```python
from build123d import *

# Parameters (mm, degrees)
BOSS_EXTRUDE1_DEPTH = 31.75
SKETCH2_R           = 3.175
CUT_EXTRUDE1_DEPTH  = 4.175
SKETCH3_R           = 3.175
CUT_EXTRUDE2_DEPTH  = 4.175


with BuildPart() as part:
    # Sketch1 → Boss-Extrude1 (new body)
    with BuildSketch(Plane.XY):
        Polygon((0, 0), (0, 25.4), (3.175, 25.4), (3.175, 3.175), (38.1, 3.175), (38.1, 0), align=None)
    extrude(amount=BOSS_EXTRUDE1_DEPTH)

    # Sketch2 → Cut-Extrude1 (cut, through all)
    with BuildSketch(Plane(origin=(0, 3.175, 0), x_dir=(1, 0, 0), z_dir=(0, 1, 0))):
        with Locations((31.9786, -6.35)):
            Circle(SKETCH2_R)
        with Locations((31.9786, -25.4)):
            Circle(SKETCH2_R)
    extrude(amount=-CUT_EXTRUDE1_DEPTH, mode=Mode.SUBTRACT)

    # Sketch3 → Cut-Extrude2 (cut, through all)
    with BuildSketch(Plane(origin=(3.175, 0, 0), x_dir=(0, 0, -1), z_dir=(1, 0, 0))):
        with Locations((-25.4, 15.875)):
            Circle(SKETCH3_R)
        with Locations((-6.35, 15.875)):
            Circle(SKETCH3_R)
    extrude(amount=-CUT_EXTRUDE2_DEPTH, mode=Mode.SUBTRACT)


solid = part.part
```
Check sheet for the modelled part. Datum: model origin and axes. Units: mm. A direction names the side the tool comes from. Round coordinates to 2 decimals unless told otherwise and drop trailing zeros. Order: outer loops, then holes, each group sorted by start corner. A loop starts at its lowest first (then second) coordinate and runs counter-clockwise, first axis right, second up.
1) Tool access check on faces 5 (the flat face through (2, 25.4, 16)), 6 (the flat face through (3.175, 14, 16)). Record the directions out of +Z, -Z, +X, -X, +Y, -Y that give a thin tool (end or side, any length) a straight path to the whole face; none if there is none.
2) Section check C-C (y = 17). Record the boundary of the cut face in (x, z) (3 decimals), and give its area (3 significant figures).
3) Go/stop test with flat-tipped pins: pin 1 Ø6 at (y, z) = (5.5, 7) entering from -X; pin 2 Ø16 at (x, z) = (26, 20) entering from +Y (3 decimals); pin 3 Ø11 at (y, z) = (17, 22) entering from +X (3 decimals). Record where each tip stops, or that it passes through.
4) Section check D-D (z = 21.5). Record the boundary of the cut face in (x, y) (3 decimals).
5) Section check B-B (x = 30.5). Record the boundary of the cut face in (y, z) (3 decimals), and give its area (3 significant figures).
6) Section check A-A (z = 6.35). Record the boundary of the cut face in (x, y) (3 decimals), and give its area (3 significant figures).
7) Mould release check, pull along X, two halves, no side actions. Record for faces 1 (the cylindrical face through (34.91, 1.61, 7.57)), 2 (the flat face through (38.1, 2, 16)), 3 (the cylindrical face through (33.685, 1.61, 22.723)), 4 (the flat face through (20, 3.175, 16)): +X half, -X half, draft (parallel to the pull), parting line (faces both ways), or undercut.
8) Scan lines: line 1 (X direction, y = 1.05, z = 6.35); line 2 (Y direction, x = 1.35, z = 25.4); line 3 (X direction, y = 6.5, z = 18) (3 decimals). Record each from-to range of solid material in increasing order.
Result:
1. face 5: +Z, -Z, +X, -X, +Y
1. face 6: +Z, -Z, +X, +Y
2. outline: (0, 0) - (3.175, 0) - (3.175, 3.381) - (0, 3.381) - close; (0, 9.319) - (3.175, 9.319) - (3.175, 22.431) - (0, 22.431) - close; (0, 28.369) - (3.175, 28.369) - (3.175, 31.75) - (0, 31.75) - close
2. area: 63.1 mm2
3. pin 1: stops at x = 0
3. pin 2: stops at y = 3.175
3. pin 3: stops at x = 3.175
4. outline: (0, 0) - (38.1, 0) - (38.1, 3.175) - (3.175, 3.175) - (3.175, 25.4) - (0, 25.4) - close
5. outline: (0, 0) - (3.175, 0) - (3.175, 3.54) - (0, 3.54) - close; (0, 9.16) - (3.175, 9.16) - (3.175, 22.59) - (0, 22.59) - close; (0, 28.21) - (3.175, 28.21) - (3.175, 31.75) - (0, 31.75) - close
5. area: 65.1 mm2
6. outline: (0, 0) - (28.804, 0) - (28.804, 3.175) - (3.175, 3.175) - (3.175, 12.7) - (0, 12.7) - close; (0, 19.05) - (3.175, 19.05) - (3.175, 25.4) - (0, 25.4) - close; (35.154, 0) - (38.1, 0) - (38.1, 3.175) - (35.154, 3.175) - close
6. area: 151 mm2
7. face 1: undercut
7. face 2: +X half
7. face 3: undercut
7. face 4: draft
8. line 1: x = 0 to 28.8, 35.15 to 38.1
8. line 2: y = 0 to 12.7, 19.05 to 25.4
8. line 3: x = 0 to 3.175
